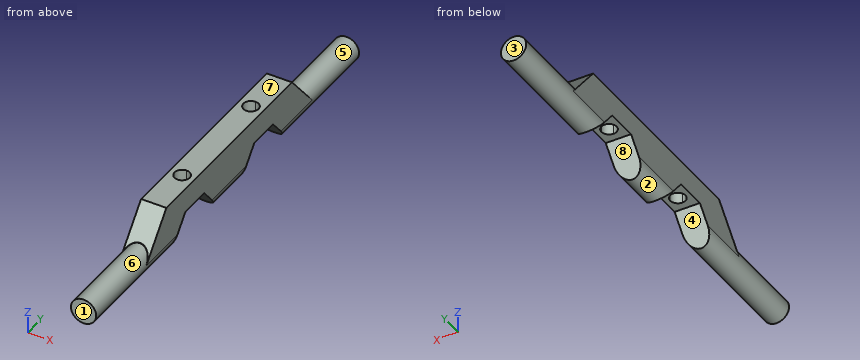
from build123d import *

# Parameters (mm, degrees)
F0_R      = 2.5
F1_DEPTH  = 85
F3_DEPTH  = 2.5
F5_DEPTH  = 25
F8_DEPTH  = 25
F9_DEPTH  = 25
F11_DEPTH = 25
F14_DEPTH = 102
F16_REACH = 96.5783545855
F18_REACH = 97.7333268634
F19_DEPTH = 1


with BuildPart() as f1:
    # F0 (on Front) → F1 (new body)
    with BuildSketch(Plane.XZ):
        Circle(F0_R)
    extrude(amount=F1_DEPTH)

    # F2 (on Right) → F3 (join, symmetric)
    with BuildSketch(Plane.YZ):
        Polygon((-69, 0), (-16, 0), (-22.4278760969, 7.6604444312), (-62.5721239031, 7.6604444312), align=None)
    extrude(amount=F3_DEPTH, both=True)

    # F4 (on face) → F5 (cut)
    with BuildSketch(Plane(origin=(-2.5, 0, 0), x_dir=(0, -1, 0), z_dir=(-1, 0, 0))):
        Polygon((56.5, 3), (53.5, 3), (50.5, 3), (44.1691353238, -4.5448307221), (62.8308646762, -4.5448307221), align=None)
        Polygon((40.8308646762, -4.5448307221), (34.5, 3), (31.5, 3), (28.5, 3), (22.1691353238, -4.5448307221), align=None)
    extrude(amount=-F5_DEPTH, mode=Mode.SUBTRACT)

    # F7 (on face) → F8 (cut)
    with BuildSketch(Plane(origin=(-2.5, 0, 0), x_dir=(0, -1, 0), z_dir=(-1, 0, 0))):
        Polygon((19.9172031134, 7.5), (22.2932472338, 7.5), (22.4278760969, 7.6604444312), (62.5721239031, 7.6604444312), (62.7067527662, 7.5), (66.5233954787, 7.5), (66.5233954787, 10.3880958632), (19.9172031134, 10.3880958632), align=None)
    extrude(amount=-F8_DEPTH, mode=Mode.SUBTRACT)

    # F6 (on face) → F9 (cut)
    with BuildSketch(Plane(origin=(0, 0, 3), x_dir=(1, 0, 0), z_dir=(0, 0, -1))):
        with BuildLine():
            ThreePointArc((1.45, 53.5), (1.0253048327, 54.5253048327), (0, 54.95))
            Line((0, 54.95), (0, 52.05))
            ThreePointArc((0, 52.05), (1.0253048327, 52.4746951673), (1.45, 53.5))
        make_face()
        with BuildLine():
            Line((0, 52.05), (0, 54.95))
            ThreePointArc((0, 54.95), (-1.45, 53.5), (0, 52.05))
        make_face()
    extrude(amount=-F9_DEPTH, mode=Mode.SUBTRACT)

    # F10 (on face) → F11 (cut)
    with BuildSketch(Plane(origin=(0, 0, 3), x_dir=(1, 0, 0), z_dir=(0, 0, -1))):
        with BuildLine():
            ThreePointArc((1.45, 31.5), (1.0253048327, 32.5253048327), (0, 32.95))
            Line((0, 32.95), (0, 30.05))
            ThreePointArc((0, 30.05), (1.0253048327, 30.4746951673), (1.45, 31.5))
        make_face()
        with BuildLine():
            Line((0, 30.05), (0, 32.95))
            ThreePointArc((0, 32.95), (-1.45, 31.5), (0, 30.05))
        make_face()
    extrude(amount=-F11_DEPTH, mode=Mode.SUBTRACT)

    # F13 (on face) → F14 (cut)
    with BuildSketch(Plane.XZ.offset(85)):
        with BuildLine():
            ThreePointArc((2.4, 0), (0, -2.4), (-2.4, 0))
            Line((-2.4, 0), (-2.4, 9.7710704431))
            Line((-2.4, 9.7710704431), (-6.1972029507, 9.7710704431))
            Line((-6.1972029507, 9.7710704431), (-6.1972029507, -5.7614380494))
            Line((-6.1972029507, -5.7614380494), (5.5722752586, -5.7614380494))
            Line((5.5722752586, -5.7614380494), (5.5722752586, 8.8547384366))
            Line((5.5722752586, 8.8547384366), (2.4, 9.1607915238))
            Line((2.4, 9.1607915238), (2.4, 0))
        make_face()
    extrude(amount=-F14_DEPTH, mode=Mode.SUBTRACT)

    f16_end = Plane(origin=(0, -64.9529870595, 4.8230422111), x_dir=(0, -0.6427876097, -0.7660444431), z_dir=(0, -0.7660444431, 0.6427876097))
    # F15 (on face) → F16 (cut, up to a plane its end follows)
    with BuildSketch(Plane.XZ.offset(85)):
        with BuildLine():
            ThreePointArc((-2.4, 0), (0, 2.4), (2.4, 0))
            Line((2.4, 0), (4.8319334164, 0))
            Line((4.8319334164, 0), (4.1808704846, 8.0774491653))
            Line((4.1808704846, 8.0774491653), (-2.9383567162, 8.0774491653))
            Line((-2.9383567162, 8.0774491653), (-3.4620375372, 0))
            Line((-3.4620375372, 0), (-2.4, 0))
        make_face()
    f16_long = extrude(amount=-F16_REACH, mode=Mode.PRIVATE)
    add(split(f16_long, bisect_by=f16_end, keep=Keep.TOP, mode=Mode.PRIVATE), mode=Mode.SUBTRACT)

    f18_end = Plane(origin=(0, -20.0470129405, 4.8230422111), x_dir=(0, -0.6427876097, 0.7660444431), z_dir=(0, 0.7660444431, 0.6427876097))
    # F17 (on face) → F18 (cut, up to a plane its end follows)
    with BuildSketch(Plane(origin=(0, 0, 0), x_dir=(-1, 0, 0), z_dir=(0, 1, 0))):
        with BuildLine():
            ThreePointArc((-2.4, 0), (0, 2.4), (2.4, 0))
            Line((2.4, 0), (3.9089121856, 0))
            Line((3.9089121856, 0), (4.3247276917, 8.6870230734))
            Line((4.3247276917, 8.6870230734), (-4.9837511033, 8.3660408854))
            Line((-4.9837511033, 8.3660408854), (-3.4170385916, 0))
            Line((-3.4170385916, 0), (-2.4, 0))
        make_face()
    f18_long = extrude(amount=-F18_REACH, mode=Mode.PRIVATE)
    add(split(f18_long, bisect_by=f18_end, keep=Keep.TOP, mode=Mode.PRIVATE), mode=Mode.SUBTRACT)

    # F19 (cut): a face of the model
    f19_faces = [f1.faces().sort_by_distance(p)[0] for p in [
        (0, 0, 0),
    ]]
    extrude(f19_faces, amount=-F19_DEPTH, mode=Mode.SUBTRACT)


solid = f1.part
For this review, take the finished solid that the model builds, in its own axes (mm). Face numbers are marked on the shaded views. A direction names the side the tool comes from. Give positions to 0.01 mm unless a question says otherwise; leave off trailing zeros. Loops run counter-clockwise (first coordinate to the right, second up) from the corner with the lowest first, then second, coordinate; pieces in that order, holes last. Notation, with made-up numbers: (52.5, -10.5) - (98.5, -10.5) arc R12 ccw to (98.5, -3.5) - close; hole circle Ø1 at (56, 54.25). An arc over 180 degrees is marked (long way). Write each question's results on one line, items separated by ' | '.
(1) Take a section at B-B (y = -73). Give the boundary of the cut face in (x, z), then the cut area to 3 significant figures.
Conclusion:
outline: circle Ø4.8 at (0, 0) | area: 18.1 mm^2
(2) Take a section at A-A (z = 5.5). Give the boundary of the cut face in (x, y).
Conclusion:
outline: (-2.4, -64.38) - (2.4, -64.38) - (2.4, -20.62) - (-2.4, -20.62) - close; hole circle Ø2.9 at (0, -53.5); hole circle Ø2.9 at (0, -31.5)
(3) Draft analysis for pull direction Y (two halves, no side actions). For the marked faces 1, 2, 3 and 4, state which applies: +Y half, -Y half, draft (parallel to the pull), parting line (faces both ways), or undercut.
Conclusion:
face 1: -Y half | face 2: draft | face 3: +Y half | face 4: undercut
(4) For line 1 along Y through (x, z) = (-0.8, 6.5); line 2 along Y through (x, z) = (0.45, 6); line 3 along Z through (x, y) = (2.15, -31.5), list the stretches that pass through material, from the lowest coordinate up.
Conclusion:
line 1: -63.55 to -54.71, -52.29 to -32.71, -30.29 to -21.45 | line 2: -63.97 to -54.88, -52.12 to -32.88, -30.12 to -21.03 | line 3: 3 to 7.66
(5) For pin 1 Ø1.5 at (x, y) = (-1, -33.5) entering from -Z; pin 2 Ø2 at (x, y) = (1.5, -12) entering from -Z, all flat-tipped, find the tip position at first contact; note any pin that passes through.
Conclusion:
pin 1: z = 3 | pin 2: z = -2.35
(6) For the marked faces 5, 6, 7 and 8, list the 3-axis set-ups (+Z, -Z, +X, -X, +Y, -Y) from which the entire face can be reached by the end or side of a thin tool; tool diameter is ignored.
Conclusion:
face 5: +Y | face 6: -Y | face 7: +Z, +X, -X, +Y, -Y | face 8: -Z, +X, -X
